```python
from build123d import *

# Parameters (mm, degrees)
EXTRUDE_4_DEPTH     = 3
SKETCH_5_R          = 3.5
EXTRUDE_6_DEPTH     = 27.5
SKETCH_8_R          = 1.5
CUT_EXTRUDE_1_DEPTH = 10
SKETCH_10_W         = 2
SKETCH_10_H         = 23.5
CUT_EXTRUDE_2_DEPTH = 5
FILLET_1_R          = 0.5


with BuildPart() as part:
    # 草图4 → 凸台-拉伸4 (new body)
    with BuildSketch(Plane.XY):
        with BuildLine():
            ThreePointArc((8.536063079, 0.007574004), (7.787120491, 0.307636704), (6.986931627, 0.410837493))
            ThreePointArc((6.986931627, 0.410837493), (6.952112765, 0.808782481), (6.894647301, 1.204092849))
            ThreePointArc((6.894647301, 1.204092849), (7.649774364, 1.488233206), (8.309831075, 1.95221355))
            ThreePointArc((8.309831075, 1.95221355), (8.220185959, 2.300646222), (8.115937918, 2.644991862))
            ThreePointArc((8.115937918, 2.644991862), (7.310926717, 2.698932461), (6.518011085, 2.549810286))
            ThreePointArc((6.518011085, 2.549810286), (6.361924616, 2.91751884), (6.18511409, 3.275723537))
            ThreePointArc((6.18511409, 3.275723537), (6.815478405, 3.77930417), (7.29985183, 4.424544441))
            ThreePointArc((7.29985183, 4.424544441), (7.106922641, 4.72822174), (6.901368208, 5.023499488))
            ThreePointArc((6.901368208, 5.023499488), (6.119088497, 4.826037904), (5.411062205, 4.439189883))
            ThreePointArc((5.411062205, 4.439189883), (5.148986959, 4.740668128), (4.870138818, 5.026703581))
            ThreePointArc((4.870138818, 5.026703581), (5.314035933, 5.70043051), (5.575312226, 6.463770094))
            ThreePointArc((5.575312226, 6.463770094), (5.297984218, 6.69296597), (5.011244492, 6.910271984))
            ThreePointArc((5.011244492, 6.910271984), (4.328271261, 6.480737132), (3.774440855, 5.894030644))
            ThreePointArc((3.774440855, 5.894030644), (3.432030584, 6.099767788), (3.078440426, 6.285634856))
            ThreePointArc((3.078440426, 6.285634856), (3.292418599, 7.063558994), (3.305022217, 7.870276894))
            ThreePointArc((3.305022217, 7.870276894), (2.970442186, 8.002556058), (2.63058525, 8.12061891))
            ThreePointArc((2.63058525, 8.12061891), (2.113772678, 7.501056656), (1.768350936, 6.77192262))
            ThreePointArc((1.768350936, 6.77192262), (1.379123142, 6.861779679), (0.985402836, 6.929284397))
            ThreePointArc((0.985402836, 6.929284397), (0.948516393, 7.735257109), (0.711213605, 8.506386157))
            ThreePointArc((0.711213605, 8.506386157), (0.352132577, 8.528800203), (-0.007574004, 8.536063079))
            ThreePointArc((-0.007574004, 8.536063079), (-0.307636703, 7.787120491), (-0.410837493, 6.986931627))
            ThreePointArc((-0.410837493, 6.986931627), (-0.808782481, 6.952112765), (-1.204092849, 6.894647301))
            ThreePointArc((-1.204092849, 6.894647301), (-1.488233206, 7.649774364), (-1.95221355, 8.309831075))
            ThreePointArc((-1.95221355, 8.309831075), (-2.300646222, 8.220185959), (-2.644991862, 8.115937918))
            ThreePointArc((-2.644991862, 8.115937918), (-2.698932461, 7.310926717), (-2.549810286, 6.518011085))
            ThreePointArc((-2.549810286, 6.518011085), (-2.91751884, 6.361924616), (-3.275723537, 6.18511409))
            ThreePointArc((-3.275723537, 6.18511409), (-3.77930417, 6.815478405), (-4.424544441, 7.29985183))
            ThreePointArc((-4.424544441, 7.29985183), (-4.72822174, 7.106922641), (-5.023499488, 6.901368208))
            ThreePointArc((-5.023499488, 6.901368208), (-4.826037904, 6.119088497), (-4.439189882, 5.411062205))
            ThreePointArc((-4.439189882, 5.411062205), (-4.740668128, 5.148986959), (-5.026703581, 4.870138818))
            ThreePointArc((-5.026703581, 4.870138818), (-5.70043051, 5.314035933), (-6.463770094, 5.575312226))
            ThreePointArc((-6.463770094, 5.575312226), (-6.69296597, 5.297984218), (-6.910271984, 5.011244492))
            ThreePointArc((-6.910271984, 5.011244492), (-6.480737132, 4.328271262), (-5.894030644, 3.774440855))
            ThreePointArc((-5.894030644, 3.774440855), (-6.099767788, 3.432030584), (-6.285634856, 3.078440426))
            ThreePointArc((-6.285634856, 3.078440426), (-7.063558994, 3.292418599), (-7.870276894, 3.305022217))
            ThreePointArc((-7.870276894, 3.305022217), (-8.002556058, 2.970442186), (-8.12061891, 2.63058525))
            ThreePointArc((-8.12061891, 2.63058525), (-7.501056656, 2.113772678), (-6.77192262, 1.768350936))
            ThreePointArc((-6.77192262, 1.768350936), (-6.861779679, 1.379123142), (-6.929284397, 0.985402836))
            ThreePointArc((-6.929284397, 0.985402836), (-7.735257109, 0.948516393), (-8.506386157, 0.711213605))
            ThreePointArc((-8.506386157, 0.711213605), (-8.528800203, 0.352132577), (-8.536063079, -0.007574004))
            ThreePointArc((-8.536063079, -0.007574004), (-7.787120492, -0.307636703), (-6.986931627, -0.410837493))
            ThreePointArc((-6.986931627, -0.410837493), (-6.952112765, -0.808782481), (-6.894647301, -1.204092849))
            ThreePointArc((-6.894647301, -1.204092849), (-7.649774364, -1.488233206), (-8.309831076, -1.95221355))
            ThreePointArc((-8.309831076, -1.95221355), (-8.220185959, -2.300646222), (-8.115937918, -2.644991862))
            ThreePointArc((-8.115937918, -2.644991862), (-7.310926717, -2.698932461), (-6.518011085, -2.549810286))
            ThreePointArc((-6.518011085, -2.549810286), (-6.361924616, -2.91751884), (-6.18511409, -3.275723537))
            ThreePointArc((-6.18511409, -3.275723537), (-6.815478405, -3.77930417), (-7.29985183, -4.424544441))
            ThreePointArc((-7.29985183, -4.424544441), (-7.106922641, -4.72822174), (-6.901368208, -5.023499488))
            ThreePointArc((-6.901368208, -5.023499488), (-6.119088498, -4.826037904), (-5.411062205, -4.439189883))
            ThreePointArc((-5.411062205, -4.439189883), (-5.148986959, -4.740668128), (-4.870138818, -5.026703582))
            ThreePointArc((-4.870138818, -5.026703582), (-5.314035933, -5.70043051), (-5.575312227, -6.463770094))
            ThreePointArc((-5.575312227, -6.463770094), (-5.297984218, -6.69296597), (-5.011244492, -6.910271984))
            ThreePointArc((-5.011244492, -6.910271984), (-4.328271262, -6.480737132), (-3.774440855, -5.894030644))
            ThreePointArc((-3.774440855, -5.894030644), (-3.432030584, -6.099767789), (-3.078440426, -6.285634856))
            ThreePointArc((-3.078440426, -6.285634856), (-3.292418599, -7.063558994), (-3.305022217, -7.870276894))
            ThreePointArc((-3.305022217, -7.870276894), (-2.970442186, -8.002556058), (-2.63058525, -8.12061891))
            ThreePointArc((-2.63058525, -8.12061891), (-2.113772678, -7.501056656), (-1.768350936, -6.77192262))
            ThreePointArc((-1.768350936, -6.77192262), (-1.379123142, -6.861779679), (-0.985402836, -6.929284397))
            ThreePointArc((-0.985402836, -6.929284397), (-0.948516393, -7.735257109), (-0.711213605, -8.506386157))
            ThreePointArc((-0.711213605, -8.506386157), (-0.352132577, -8.528800203), (0.007574004, -8.536063079))
            ThreePointArc((0.007574004, -8.536063079), (0.307636704, -7.787120491), (0.410837493, -6.986931627))
            ThreePointArc((0.410837493, -6.986931627), (0.808782481, -6.952112765), (1.204092849, -6.894647301))
            ThreePointArc((1.204092849, -6.894647301), (1.488233206, -7.649774364), (1.95221355, -8.309831075))
            ThreePointArc((1.95221355, -8.309831075), (2.300646222, -8.220185959), (2.644991862, -8.115937918))
            ThreePointArc((2.644991862, -8.115937918), (2.698932461, -7.310926717), (2.549810286, -6.518011085))
            ThreePointArc((2.549810286, -6.518011085), (2.91751884, -6.361924616), (3.275723537, -6.18511409))
            ThreePointArc((3.275723537, -6.18511409), (3.77930417, -6.815478405), (4.424544441, -7.29985183))
            ThreePointArc((4.424544441, -7.29985183), (4.72822174, -7.106922641), (5.023499488, -6.901368208))
            ThreePointArc((5.023499488, -6.901368208), (4.826037904, -6.119088497), (4.439189883, -5.411062205))
            ThreePointArc((4.439189883, -5.411062205), (4.740668128, -5.148986959), (5.026703582, -4.870138818))
            ThreePointArc((5.026703582, -4.870138818), (5.70043051, -5.314035933), (6.463770094, -5.575312226))
            ThreePointArc((6.463770094, -5.575312226), (6.69296597, -5.297984218), (6.910271984, -5.011244492))
            ThreePointArc((6.910271984, -5.011244492), (6.480737132, -4.328271261), (5.894030644, -3.774440855))
            ThreePointArc((5.894030644, -3.774440855), (6.099767788, -3.432030584), (6.285634856, -3.078440425))
            ThreePointArc((6.285634856, -3.078440425), (7.063558994, -3.292418599), (7.870276894, -3.305022217))
            ThreePointArc((7.870276894, -3.305022217), (8.002556058, -2.970442186), (8.12061891, -2.63058525))
            ThreePointArc((8.12061891, -2.63058525), (7.501056656, -2.113772678), (6.77192262, -1.768350936))
            ThreePointArc((6.77192262, -1.768350936), (6.861779679, -1.379123142), (6.929284397, -0.985402836))
            ThreePointArc((6.929284397, -0.985402836), (7.735257109, -0.948516393), (8.506386157, -0.711213605))
            ThreePointArc((8.506386157, -0.711213605), (8.528643141, -0.355916321), (8.536066439, 0))
            ThreePointArc((8.536066439, 0), (8.536065599, 0.003787002), (8.536063079, 0.007574004))
        make_face()
    extrude(amount=EXTRUDE_4_DEPTH)

    # 草图5 → 凸台-拉伸6 (add)
    with BuildSketch(Plane.XY.offset(3)):
        Circle(SKETCH_5_R)
    extrude(amount=EXTRUDE_6_DEPTH)

    # 草图8 → 切除-拉伸1 (cut)
    with BuildSketch(Plane.XY.offset(30.5)):
        Circle(SKETCH_8_R)
    extrude(amount=-CUT_EXTRUDE_1_DEPTH, mode=Mode.SUBTRACT)

    # 草图10 → 切除-拉伸2 (cut, symmetric)
    with BuildSketch(Plane(origin=(0, 0, 0), x_dir=(1, 0, 0), z_dir=(0, 1, 0))):
        with Locations((0, -16.75)):
            Rectangle(SKETCH_10_W, SKETCH_10_H)
    extrude(amount=CUT_EXTRUDE_2_DEPTH, both=True, mode=Mode.SUBTRACT)

    # 圆角1
    fillet_1_edges = [part.edges().sort_by_distance(p)[0] for p in [
        (-3.5, 0, 30.5),
    ]]
    fillet(fillet_1_edges, radius=FILLET_1_R)


solid = part.part
```
Input: part model. Units: mm. Frame: model coordinates. A direction names the side the tool comes from. Give positions to 0.01 mm unless a question says otherwise; leave off trailing zeros. Order: outer loops, then holes, each group sorted by start corner. A loop starts at its lowest first (then second) coordinate and runs counter-clockwise, first axis right, second up. Notation, with made-up numbers: (52, 85.5) - (91, 85.5) arc R26 cw to (91, 117.5) - close; hole circle Ø1 at (53, -8). An arc over 180 degrees is marked (long way). Use a Markdown table: item, result.
(1) Section query A-A (z = 27). Output: boundary loops of the cut face in (x, y).
Computed values:
| item | result |
|---|---|
| outline | (-1, -3.35) - (-1, -1.12) arc R1.5 cw to (-1, 1.12) - (-1, 3.35) arc R3.5 ccw to start; (1, -3.35) arc R3.5 ccw to (1, 3.35) - (1, 1.12) arc R1.5 cw to (1, -1.12) - close |
(2) Pin query (flat end, axial travel): pin 1 (4 mm diameter, centred on y = -3, z = 26, fed in from +X); pin 2 (6 mm diameter, centred on x = 6, z = 15.5, fed in from +Y); pin 3 (0.6 mm diameter, centred on x = 0, y = 0.5, fed in from +Z); pin 4 (2 mm diameter, centred on y = 4.5, z = 15, fed in from -X). Return the tip coordinate at first contact, or that it passes through.
Computed values:
| item | result |
|---|---|
| pin 1 | stops at x = 3.35 |
| pin 2 | stops at y = 1.8 |
| pin 3 | stops at z = 5 |
| pin 4 | passes through |
(3) Line query: line 1 (Z direction, x = -0.5, y = -3); line 2 (Y direction, x = 0, z = 28.75); line 3 (X direction, y = 1, z = 12.5). Output: solid intervals per line, ascending. Write a range as from..to.
Computed values:
| item | result |
|---|---|
| line 1 | z = 0..5, 28.5..30.5 |
| line 2 | y = -3.5..-1.5, 1.5..3.5 |
| line 3 | x = -3.35..-1, 1..3.35 |
(4) Draft query along Z for faces 1 (the flat face through (1.3, -1.3, 30.5)), 2 (the flat face through (1, 0, 17)), 3 (the cylindrical face through (0.305, -7.798, 1.479)). Return one class per face: released by +Z, released by -Z, zero draft, split by the parting line, or undercut.
Computed values:
| item | result |
|---|---|
| face 1 | released by +Z |
| face 2 | undercut |
| face 3 | zero draft |
(5) Section query B-B (z = 18). Output: boundary loops of the cut face in (x, y).
Computed values:
| item | result |
|---|---|
| outline | (-1, -3.35) - (-1, 3.35) arc R3.5 ccw to start; (1, -3.35) arc R3.5 ccw to (1, 3.35) - close |
(6) Access query for faces 4 (the cylindrical face through (3.233, -1.341, 16.311)), 5 (the flat face through (-1, 0, 17)), 6 (the cylindrical face through (3.771, -6.808, 1.479)), 7 (the cylindrical face through (6.49, -4.34, 1.48)). Directions: +Z, -Z, +X, -X, +Y, -Y. A direction counts if a zero-diameter tool reaches every point of the face in a straight line with its end or side. Return the directions, or none.
Computed values:
| item | result |
|---|---|
| face 4 | +Z |
| face 5 | +Y, -Y |
| face 6 | +Z, -Z, -Y |
| face 7 | +Z, -Z, +X |
